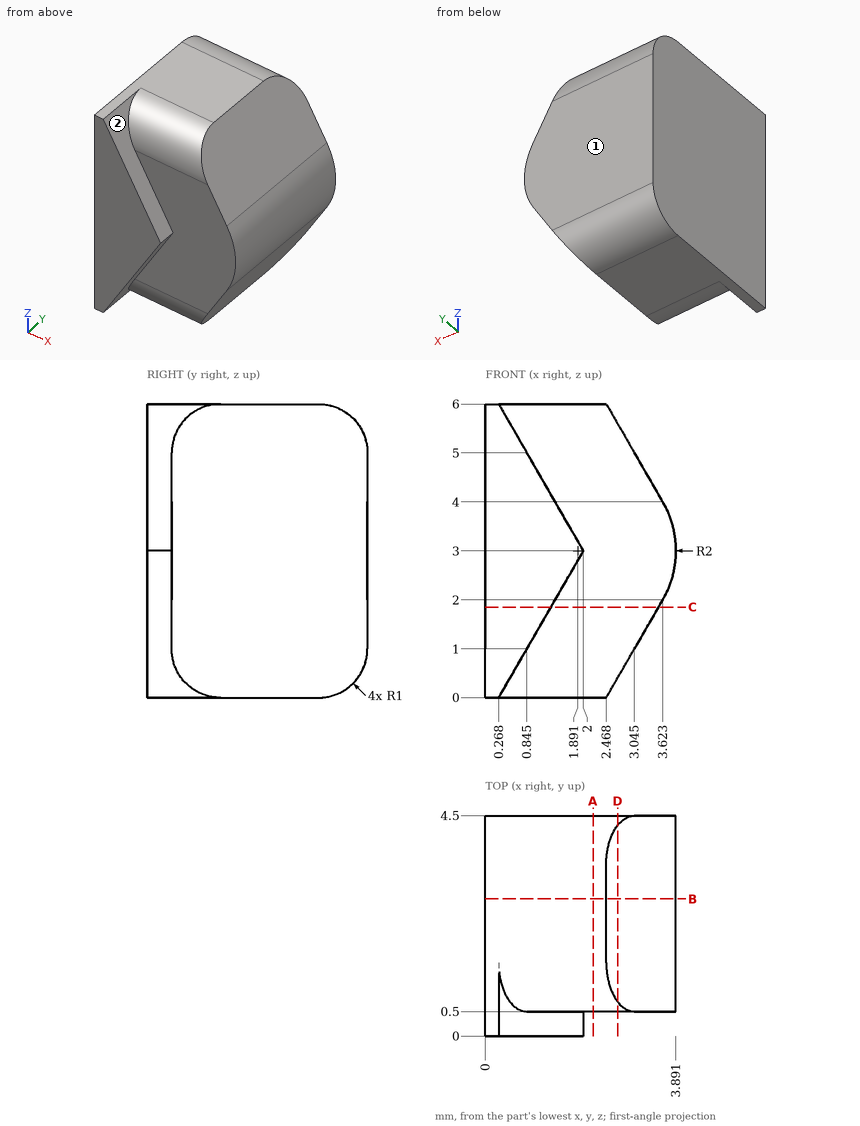
Job drawing, mm, ordinate dimensions from the low corner. One solid piece. A direction names the side the tool comes from. Give positions to 0.01 mm unless a question says otherwise; leave off trailing zeros. Loops run counter-clockwise (first coordinate to the right, second up) from the corner with the lowest first, then second, coordinate; pieces in that order, holes last. Notation, with made-up numbers: M -34,65 L -5,65 A37 cw -5,103 Z; hole C 84,60 d7. An arc over 180 degrees is marked long. Answer in a Markdown table with one row per item. Add a question column.
Item 1: Drop a flat-ended pin along its axis: P1, Ø1.5, axis at y = 2, z = 1.5, coming from the +X side (1 decimal). Give the stop position or say it passes through.
Item 2: Tool access for the marked faces 1 and 2: list every direction of +Z, -Z, +X, -X, +Y, -Y with a clear straight run to the whole face (end or side of a thin tool).
Item 3: Band-saw the part on A-A on x = 2.2. Give the cut face in (y, z).
Item 4: Band-saw the part on D-D on x = 2.7. Give the cut face in (y, z), then the cut area to 3 significant figures.
Item 5: Band-saw the part on B-B on y = 2.8. Give the cut face in (x, z), then the cut area to 3 significant figures.
Item 6: Band-saw the part on C-C on z = 1.85. Give the cut face in (x, y).
Item 7: Probe probe 1 along Y at (x, z) = (1, 0.95); probe 2 along X at (y, z) = (0.3, 5.05) (1 decimal); probe 3 along Z at (x, y) = (1.25, 0.4). List the from-to ranges inside material, lowest first.
Reply:
| question | item | result |
|---|---|---|
| 1 | P1 | stops at x = 3.7 |
| 2 | face 1 | +Z, -Z, +X, -X, +Y |
| 2 | face 2 | +Z, +X, -Y |
| 3 | outline | M 0.5,1 A1 ccw 1.5,0 L 3.5,0 A1 ccw 4.5,1 L 4.5,5 A1 ccw 3.5,6 L 1.5,6 A1 ccw 0.5,5 Z |
| 4 | outline | M 0.5,1 A1 ccw 0.7,0.4 L 4.3,0.4 A1 ccw 4.5,1 L 4.5,5 A1 ccw 4.3,5.6 L 0.7,5.6 A1 ccw 0.5,5 Z |
| 4 | area | 20.6 mm^2 |
| 5 | outline | M 0,0 L 2.47,0 L 3.62,2 A2 ccw 3.62,4 L 2.47,6 L 0,6 Z |
| 5 | area | 19.8 mm^2 |
| 6 | outline | M 0,0 L 1.34,0 L 1.34,0.5 L 3.54,0.5 L 3.54,4.5 L 0,4.5 Z |
| 7 | probe 1 | y = 0.5 to 4.5 |
| 7 | probe 2 | x = 0 to 0.8 |
| 7 | probe 3 | z = 1.7 to 4.3 |
